The listing builds one solid part. Answer for the finished solid, in the listing's coordinates (mm). Face numbers are marked on the shaded views. Give positions to 0.01 mm unless a question says otherwise; leave off trailing zeros. Order: outer loops, then holes, each group sorted by start corner. A loop starts at its lowest first (then second) coordinate and runs counter-clockwise, first axis right, second up. Notation, with made-up numbers: (-17.75, -24) -> (1.25, -24) arc R9 cw to (1.25, -7) -> close; hole circle Ø5 at (74, 70.5). An arc over 180 degrees is marked (long way). One line per question, with ' | ' between items. Start each with the question number.
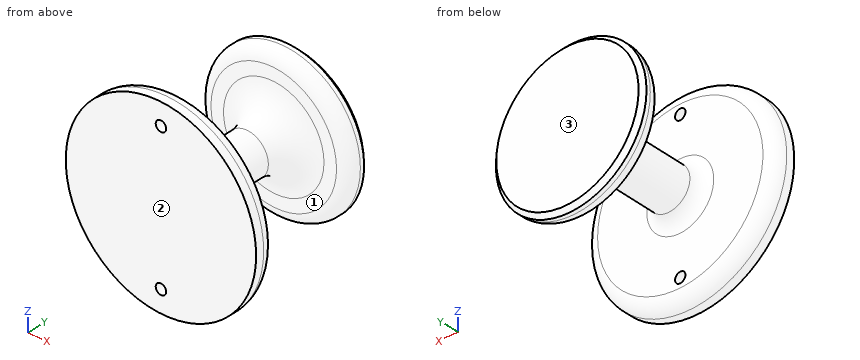
Autodesk Inventor part; units mm, degrees
ref_plane "YZ Plane" through (0, 0, 0) normal (1, 0, 0) x (0, 1, 0)
ref_plane "XZ Plane" through (0, 0, 0) normal (0, 1, 0) x (-1, 0, 0)
ref_plane "XY Plane" through (0, 0, 0) normal (0, 0, 1) x (1, 0, 0)
sketch "Sketch2" plane through (0, 0, 0) normal (0, 0, 1) x (1, 0, 0)
  line L0 (0, 0) -> (22.75, 0)
  line L1 (0, 0) -> (0, 35)
  line L2 (0, 35) -> (18, 35)
  line L3 (18, 35) -> (18, 30)
  line L4 (18, 30) -> (5, 30)
  line L5 (5, 30) -> (5, 5)
  line L6 (5, 5) -> (22.75, 5)
  line L7 (22.75, 5) -> (22.75, 0)
  dimension "d3" = 22.75
  dimension "d4" = 35
  dimension "d5" = 18
  dimension "d6" = 5
  dimension "d23" = 5
  dimension "d24" = 25
  dimension "d26" = 5
revolve "Revolution1" add sketch "Sketch2" angle 360 about axis through (0, 0, 0) along (0, 1, 0)
fillet "Fillet1" radius 3 3 edges at (-5, 5, 0) (-18, 30, 0) (-22.75, 5, 0)
chamfer "Chamfer1" distance 1 angle 45 1 edges at (-18, 35, 0)
sketch "Sketch3" plane through (0, 0, 0) normal (0, -1, 0) x (1, 0, 0)
  line L0 (0, 0) -> (0, -17.5)
  line L1 (0, 0) -> (0, 17.5)
  dimension "d14" = 17.5
  dimension "d15" = 17.5
hole "Hole1" at (0, 0, 17.5) at (0, 0, -17.5) direction (0, 1, 0) diameter 2.5 depth 5
fillet "Fillet2" radius 7 1 edges at (-5, 30, 0)
properties part number "holding_socket"
(1) The part is cut by section C-C on y = 22. Determine the outline of the cut face in (x, z), plus the area to 3 significant figures.
(2) Consider line 1 (Y direction, x = 13.5, z = 6); line 2 (Z direction, x = 0, y = 2.8); line 3 (Z direction, x = 0, y = 4.05). Determine where each line is inside the solid, lowest interval first.
(3) The part is cut by section B-B on z = 0. Determine the outline of the cut face in (x, y).
(4) The part is cut by section D-D on y = 27.5. Determine the outline of the cut face in (x, z).
(5) Given P1, Ø6, axis at x = -11.5, z = -5.5, coming from the -Y side; P2, Ø10, axis at x = 4.5, y = 19.5, coming from the -Z side; P3, Ø8, axis at y = 13, z = 7.5, coming from the -X side; P4, Ø5, axis at x = 0.5, y = 21, coming from the +Z side, each flat-ended and moving along its own axis, determine where each tip first touches the part or whether it passes through.
(6) The part is cut by section A-A on x = 0. State how many separate pieces and enclosed holes the cut face has, plus the area to 3 significant figures.
(7) Determine the mould class of the marked faces 1, 2 and 3 for opening direction Y: pulls with the +Y half, pulls with the -Y half, needs draft (parallel to the pull), parting line crosses it, or undercut.
Result sheet:
1) outline: circle Ø10 at (0, 0) | area: 78.5 mm^2
2) line 1: y = 0 to 5, 30 to 35 | line 2: z = -22.64 to -18.75, -16.25 to 16.25, 18.75 to 22.64 | line 3: z = -21.94 to -18.75, -16.25 to 16.25, 18.75 to 21.94
3) outline: (-22.75, 0) -> (22.75, 0) -> (22.75, 2) arc R3 ccw to (19.75, 5) -> (8, 5) arc R3 cw to (5, 8) -> (5, 23) arc R7 cw to (12, 30) -> (15, 30) arc R3 ccw to (18, 33) -> (18, 34) -> (17, 35) -> (-17, 35) -> (-18, 34) -> (-18, 33) arc R3 ccw to (-15, 30) -> (-12, 30) arc R7 cw to (-5, 23) -> (-5, 8) arc R3 cw to (-8, 5) -> (-19.75, 5) arc R3 ccw to (-22.75, 2) -> close
4) outline: circle Ø13.28 at (0, 0)
5) P1: stops at y = 0 | P2: stops at z = -5 | P3: stops at x = -3.57 | P4: stops at z = 5.01
6) separate pieces: 3 | enclosed holes: 0 | area: 649 mm^2
7) face 1: undercut | face 2: pulls with the -Y half | face 3: pulls with the +Y half
